Design review of the part built by this model. Coordinates are the model's own, in mm. Face numbers are marked on the shaded views. A direction names the side the tool comes from. Round coordinates to 2 decimals unless told otherwise and drop trailing zeros. Write each loop counter-clockwise with the first axis right and the second up, starting at its lowest first coordinate (ties: lowest second). Pieces come first, ordered by that corner, then holes. Notation, with made-up numbers: (32, 75) -> (60, 75) arc R21 cw to (60, 80) -> close; hole circle Ø11 at (84, 13). An arc over 180 degrees is marked (long way). Write item = value, one per line. Start each with the question number.
Item 1: For pin 1 Ø5 at (y, z) = (5, 4.5) entering from +X; pin 2 Ø6 at (x, y) = (5, 16) entering from -Z, all flat-tipped, find the tip position at first contact; note any pin that passes through.
Item 2: Add section B-B, the plane y = 10.5. State the section outline as (x, z) points.
Item 3: Add section C-C, the plane z = -0.75. State the section outline as (x, y) points.
Item 4: To check wall thickness, follow L1, parallel to Y at x = -3, z = -1.75; L2, parallel to Z at x = -2.25, y = 28; L3, parallel to Z at x = 2, y = 1.5. State the ranges of each line that lie inside material, in increasing order.
Item 5: Machinability: for the marked faces 1 and 2, which of the approach directions +Z, -Z, +X, -X, +Y, -Y give a long, thin tool a straight path to every point of the face, cutting with its end or side? Answer none if there is none.
Item 6: Add section A-A, the plane x = -1.25. State the section outline as (y, z) points, then the cut area to 3 significant figures.
Item 7: Add section D-D, the plane x = -6. State the section outline as (y, z) points.
from build123d import *

# Parameters (mm, degrees)
F1_DEPTH = 3
F2_R     = 2.5
F3_DEPTH = 36


with BuildPart() as f1:
    # F0 (on Front) → F1 (new body)
    with BuildSketch(Plane.XZ):
        Polygon((-3.562627, 5.942027), (-6.92726, -0.114312), (-3.364633, -6.056339), (3.562627, -5.942027), (6.92726, 0.114312), (3.364633, 6.056339), align=None)
    extrude(amount=F1_DEPTH)

    # F2 (on face) → F3 (join)
    with BuildSketch(Plane(origin=(0, 0, 0), x_dir=(-1, 0, 0), z_dir=(0, 1, 0))):
        Circle(F2_R)
    extrude(amount=F3_DEPTH)


solid = f1.part
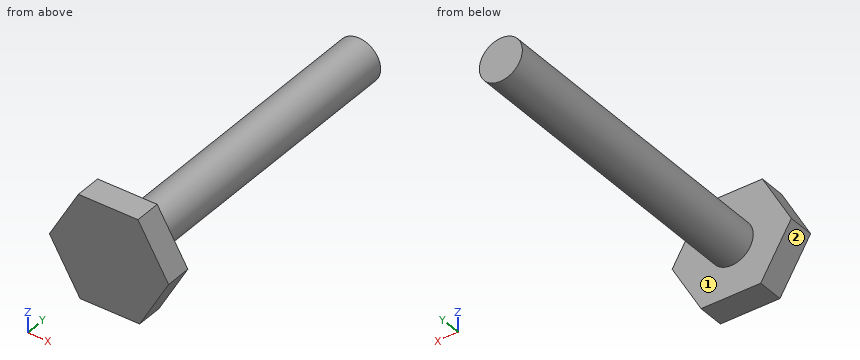
Result set:
q1.pin_1 = 1.5
q1.pin_2 = -1.5
q2.outline = circle Ø5 at (0, 0)
q3.outline = (-6.55, -3) -> (6.45, -3) -> (6.45, 0) -> (2.38, 0) -> (2.38, 36) -> (-2.38, 36) -> (-2.38, 0) -> (-6.55, 0) -> close
q4.L1 = -3 to 0
q4.L2 = -1.09 to 1.09
q4.L3 = -1.5 to 1.5
q5.face_1 = +Y
q5.face_2 = -Z, -X, +Y, -Y
q6.outline = (-3, -6.02) -> (0, -6.02) -> (0, -2.17) -> (36, -2.17) -> (36, 2.17) -> (0, 2.17) -> (0, 5.98) -> (-3, 5.98) -> close
q6.area = 192 mm²
q7.outline = (-3, -1.66) -> (0, -1.66) -> (0, 1.55) -> (-3, 1.55) -> close
